Input: part model. Units: mm. Frame: model coordinates. Face numbers are marked on the shaded views. A direction names the side the tool comes from. Coordinates: 2 decimals unless noted, no trailing zeros. Order: outer loops, then holes, each group sorted by start corner. A loop starts at its lowest first (then second) coordinate and runs counter-clockwise, first axis right, second up. Notation, with made-up numbers: M 27.25,76 L 54.25,76 A20 ccw 54.25,105 Z; hole C 61,25.5 d11. An arc over 180 degrees is marked long. One line per item, written item: value.
```python
from build123d import *

# Parameters (mm, degrees)
ESQUISSE2_R        = 15
BOSS_EXTRU_1_DEPTH = 11
ESQUISSE3_W        = 36
ESQUISSE3_H        = 32
BOSS_EXTRU_2_DEPTH = 34


with BuildPart() as part:
    # Esquisse1 → Révolution1 (revolve)
    with BuildSketch(Plane.XY, mode=Mode.PRIVATE) as r_volution1_sk:
        Polygon((0, 0), (30, 0), (30, 2), (15, 2), (15, 17), (13, 17), (13, 24), (21, 24), (21, 28), (0, 28), align=None)
    revolve(r_volution1_sk.sketch.rotate(Axis((0, 28, 0), (0, -1, 0)), 180), axis=Axis((0, 28, 0), (0, -1, 0)))

    # Esquisse2 → Boss.-Extru.1 (add)
    with BuildSketch(Plane(origin=(0, 0, 0), x_dir=(-1, 0, 0), z_dir=(0, -1, 0))):
        Circle(ESQUISSE2_R)
    extrude(amount=BOSS_EXTRU_1_DEPTH)

    # Esquisse3 → Boss.-Extru.2 (add)
    with BuildSketch(Plane(origin=(0, -11, 0), x_dir=(-1, 0, 0), z_dir=(0, -1, 0))):
        Rectangle(ESQUISSE3_W, ESQUISSE3_H)
    extrude(amount=BOSS_EXTRU_2_DEPTH)


solid = part.part
```
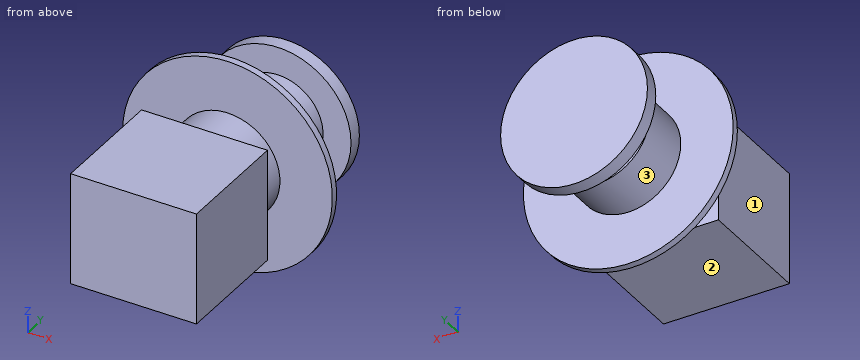
(1) Cut plane C-C on x = 0. Output: boundary loops of the cut face in (y, z).
Data:
outline: M -45,-16 L -11,-16 L -11,-15 L 0,-15 L 0,-30 L 2,-30 L 2,-15 L 17,-15 L 17,-13 L 24,-13 L 24,-21 L 28,-21 L 28,21 L 24,21 L 24,13 L 17,13 L 17,15 L 2,15 L 2,30 L 0,30 L 0,15 L -11,15 L -11,16 L -45,16 Z
(2) Access query for the marked faces 1, 2 and 3. Directions: +Z, -Z, +X, -X, +Y, -Y. A direction counts if a zero-diameter tool reaches every point of the face in a straight line with its end or side. Return the directions, or none.
Data:
face 1: +Z, -Z, -X, -Y
face 2: -Z, +X, -X, -Y
face 3: none
(3) First-contact query: pin 1 (1.5 mm diameter, centred on x = 0.5, y = 8.5, fed in from +Z); pin 2 (17 mm diameter, centred on x = -4.5, y = -31.5, fed in from -Z); pin 3 (9.5 mm diameter, centred on y = -20, z = 1, fed in from +X). Flat tips, straight axial feed; report the tip coordinate or a pass-through.
Data:
pin 1: stops at z = 15
pin 2: stops at z = -16
pin 3: stops at x = 18
(4) Ray query, line 1 (Y direction, x = -16.5, z = 2); line 2 (Y direction, x = 1.5, z = 14); line 3 (Z direction, x = 6, y = -35). Return the intervals inside material, ascending. Write a range as from..to.
Data:
line 1: y = -45..-11, 0..2, 24..28
line 2: y = -45..17, 24..28
line 3: z = -16..16
(5) Cut plane B-B on z = 0. Output: boundary loops of the cut face in (x, y), plus the area to 3 significant figures.
Data:
outline: M -30,0 L -15,0 L -15,-11 L -18,-11 L -18,-45 L 18,-45 L 18,-11 L 15,-11 L 15,0 L 30,0 L 30,2 L 15,2 L 15,17 L 13,17 L 13,24 L 21,24 L 21,28 L -21,28 L -21,24 L -13,24 L -13,17 L -15,17 L -15,2 L -30,2 Z
area: 2,470 mm2
(6) Cut plane A-A on z = 17.5. Output: boundary loops of the cut face in (x, y).
Data:
outline: M -24.37,0 L 24.37,0 L 24.37,2 L -24.37,2 Z; M -11.61,24 L 11.61,24 L 11.61,28 L -11.61,28 Z
(7) Cut plane D-D on y = -13. Output: boundary loops of the cut face in (x, z), plus the area to 3 significant figures.
Data:
outline: M -18,-16 L 18,-16 L 18,16 L -18,16 Z
area: 1,150 mm2
